```python
from build123d import *

# Parameters (mm, degrees)
SKETCH1_W            = 125
SKETCH1_H            = 125
BOSS_EXTRUDE1_DEPTH  = 15
SKETCH2_W            = 115
SKETCH2_H            = 115
CUT_EXTRUDE1_DEPTH   = 5
SKETCH3_W            = 15
SKETCH3_H            = 15
BOSS_EXTRUDE12_DEPTH = 25
SKETCH4_R            = 4.05
CUT_EXTRUDE2_DEPTH   = 25
FILLET1_R            = 7.5
FILLET1_OF_MIRROR1_R = 7.5
MIRROR2_START        = -62.5
MIRROR2_OUTLINE_R    = 4.05
MIRROR2_DEPTH        = 25
MIRROR2_START_2      = 37.5
MIRROR2_2_OUTLINE_R  = 4.05
MIRROR2_2_DEPTH      = 25


# Read off the part's stored shape, not the designer's step: Mirror2
with BuildPart() as part:
    # Sketch1 → Boss-Extrude1 (new body)
    with BuildSketch(Plane(origin=(0, 0, 0), x_dir=(1, 0, 0), z_dir=(0, 1, 0))):
        Rectangle(SKETCH1_W, SKETCH1_H)
    extrude(amount=BOSS_EXTRUDE1_DEPTH)

    # Sketch2 → Cut-Extrude1 (cut)
    with BuildSketch(Plane(origin=(0, 15, 0), x_dir=(1, 0, 0), z_dir=(0, 1, 0))):
        Rectangle(SKETCH2_W, SKETCH2_H)
    extrude(amount=-CUT_EXTRUDE1_DEPTH, mode=Mode.SUBTRACT)

    # Sketch3 → Boss-Extrude12 (add)
    with BuildSketch(Plane.ZY.offset(62.5)):
        with Locations((-70, 7.5)):
            Rectangle(SKETCH3_W, SKETCH3_H)
    boss_extrude12 = extrude(amount=-BOSS_EXTRUDE12_DEPTH)

    # Sketch4 → Cut-Extrude2 (cut)
    with BuildSketch(Plane.ZY.offset(62.5)):
        with Locations((-70, 7.5)):
            Circle(SKETCH4_R)
    cut_extrude2 = extrude(amount=-CUT_EXTRUDE2_DEPTH, mode=Mode.SUBTRACT)

    # Fillet1
    fillet1_edges = [part.edges().sort_by_distance(p)[0] for p in [
        (-50, 15, -77.5),
    ]]
    fillet(fillet1_edges, radius=FILLET1_R)

    # Mirror1: Boss-Extrude12, Cut-Extrude2 across plane
    add(boss_extrude12.mirror(Plane(origin=(0, 0, 0), x_dir=(0, 0, 1), z_dir=(1, 0, 0))))
    add(cut_extrude2.mirror(Plane(origin=(0, 0, 0), x_dir=(0, 0, 1), z_dir=(1, 0, 0))), mode=Mode.SUBTRACT)

    # Fillet1 of Mirror1
    fillet1_of_mirror1_edges = [part.edges().sort_by_distance(p)[0] for p in [
        (50, 15, -77.5),
    ]]
    fillet(fillet1_of_mirror1_edges, radius=FILLET1_OF_MIRROR1_R)

    # Mirror2 outline → Mirror2 (add)
    with BuildSketch(Plane.YZ.offset(MIRROR2_START)):
        with BuildLine():
            Line((15, 62.5), (15, 70))
            ThreePointArc((15, 70), (12.803300859, 75.303300859), (7.5, 77.5))
            Line((7.5, 77.5), (0, 77.5))
            Line((0, 77.5), (0, 62.5))
            Line((0, 62.5), (15, 62.5))
        make_face()
        with Locations((7.5, 70)):
            Circle(MIRROR2_OUTLINE_R, mode=Mode.SUBTRACT)
    extrude(amount=MIRROR2_DEPTH)

    # Mirror2 2 outline → Mirror2 2 (add)
    with BuildSketch(Plane.YZ.offset(MIRROR2_START_2)):
        with BuildLine():
            Line((15, 62.5), (15, 70))
            ThreePointArc((15, 70), (12.803300859, 75.303300859), (7.5, 77.5))
            Line((7.5, 77.5), (0, 77.5))
            Line((0, 77.5), (0, 62.5))
            Line((0, 62.5), (15, 62.5))
        make_face()
        with Locations((7.5, 70)):
            Circle(MIRROR2_2_OUTLINE_R, mode=Mode.SUBTRACT)
    extrude(amount=MIRROR2_2_DEPTH)


solid = part.part
```
The listing builds one solid part. Answer for the finished solid, in the listing's coordinates (mm). A direction names the side the tool comes from. Round coordinates to 2 decimals unless told otherwise and drop trailing zeros. Loops run counter-clockwise (first coordinate to the right, second up) from the corner with the lowest first, then second, coordinate; pieces in that order, holes last.
1) For faces 3 (the face through (-1, 7, 62.5)), 4 (the face through (57.5, 13, 1)), 5 (the face through (-37.5, 4, -67)), determine the directions among +Z, -Z, +X, -X, +Y, -Y from which every point of the face is accessible in a straight line to the end or side of a thin tool.
Outcome:
face 3: +Z, +Y, -Y
face 4: +Y
face 5: -Z, +Y, -Y
2) Given P1, Ø7.5, axis at y = 6, z = 72, coming from the -X side; P2, Ø12, axis at x = -41, z = -15, coming from the +Y side; P3, Ø5.5, axis at x = -22.5, y = 12, coming from the +Z side, each flat-ended and moving along its own axis, determine where each tip first touches the part or whether it passes through.
Outcome:
P1: stops at x = -62.5
P2: stops at y = 10
P3: stops at z = 62.5
3) For a pull along X with two mould halves and no side action, classify faces 1 (the face through (0, 15, 62)), 2 (the face through (37.5, 4, -67)) as released by +X, released by -X, zero draft, split by the parting line, or undercut.
Outcome:
face 1: zero draft
face 2: undercut
4) A cutting plane is placed at C-C on x = 3. Determine the outline of the cut face in (y, z).
Outcome:
outline: (0, -62.5) - (15, -62.5) - (15, -57.5) - (10, -57.5) - (10, 57.5) - (15, 57.5) - (15, 62.5) - (0, 62.5) - close
5) A cutting plane is placed at B-B on z = -47.5. Determine the outline of the cut face in (x, y).
Outcome:
outline: (-62.5, 0) - (62.5, 0) - (62.5, 15) - (57.5, 15) - (57.5, 10) - (-57.5, 10) - (-57.5, 15) - (-62.5, 15) - close
6) A cutting plane is placed at A-A on x = -53. Determine the outline of the cut face in (y, z).
Outcome:
outline: (0, -77.5) - (7.5, -77.5) arc R7.5 ccw to (15, -70) - (15, -57.5) - (10, -57.5) - (10, 57.5) - (15, 57.5) - (15, 70) arc R7.5 ccw to (7.5, 77.5) - (0, 77.5) - close; hole circle Ø8.1 at (7.5, -70); hole circle Ø8.1 at (7.5, 70)
7) Consider line 1 (Y direction, x = 45.5, z = -70); line 2 (X direction, y = 10.25, z = -66); line 3 (X direction, y = 10.75, z = -5). Determine where each line is inside the solid, lowest interval first.
Outcome:
line 1: y = 0 to 3.45, 11.55 to 15
line 2: x = -62.5 to -37.5, 37.5 to 62.5
line 3: x = -62.5 to -57.5, 57.5 to 62.5
